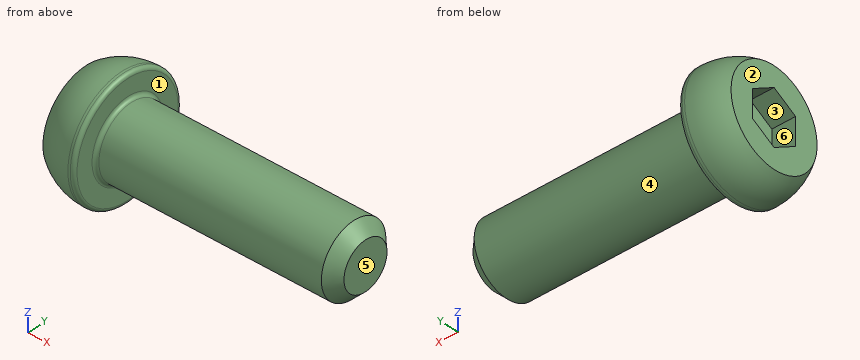
from build123d import *

# Parameters (mm, degrees)
CUT_EXTRUDE_1_DEPTH = 2
FILLET_1_R          = 0.3
CHAMFER_1_SIZE      = 1


with BuildPart() as part:
    # Эскиз1 → Повернуть1 (revolve)
    with BuildSketch(Plane.XY):
        with BuildLine():
            Line((0, 0), (0, 4))
            ThreePointArc((0, 4), (1.41886117, 4.74341649), (3, 5))
            Line((3, 5), (3.5, 5))
            Line((3.5, 5), (3.5, 3))
            Line((3.5, 3), (23.5, 3))
            Line((23.5, 3), (23.5, 0))
            Line((23.5, 0), (0, 0))
        make_face()
    revolve(axis=Axis((23.5, 0, 0), (-1, 0, 0)))

    # Эскиз2 → Вырез-Вытянуть1 (cut)
    with BuildSketch(Plane.ZY):
        Polygon((1.154700538, 2), (-1.154700538, 2), (-2.309401077, 0), (-1.154700538, -2), (1.154700538, -2), (2.309401077, 0), align=None)
    extrude(amount=-CUT_EXTRUDE_1_DEPTH, mode=Mode.SUBTRACT)

    # Скругление1
    fillet_1_edges = [part.edges().sort_by_distance(p)[0] for p in [
        (3.5, -3, 0),
        (3.5, -5, 0),
    ]]
    fillet(fillet_1_edges, radius=FILLET_1_R)

    # Фаска1
    chamfer_1_edges = [part.edges().sort_by_distance(p)[0] for p in [
        (23.5, -3, 0),
    ]]
    chamfer(chamfer_1_edges, length=CHAMFER_1_SIZE)


solid = part.part
Can you work these out from the model? Positions are in its coordinate system, mm. Face numbers are marked on the shaded views. A direction names the side the tool comes from. Coordinates: 2 decimals unless noted, no trailing zeros. Loops run counter-clockwise (first coordinate to the right, second up) from the corner with the lowest first, then second, coordinate; pieces in that order, holes last. Notation, with made-up numbers: (33.25, 62) - (60.25, 62) arc R19 cw to (60.25, 78) - close; hole circle Ø11 at (-33.75, -24). An arc over 180 degrees is marked (long way). Answer as a JSON object with one key per item and string values. Group by question number.
Item 1: On a 3-axis mill with a long thin cutter (end or side, diameter ignored), from which of +Z, -Z, +X, -X, +Y, -Y can I reach the whole of each face in a straight line? I mean the marked faces 1, 2 and 3. Say none if no direction works.
Item 2: If we section it at A-A (z = 0): List the corners of the cut face in (x, y) for me.
Item 3: If I drill on L1, parallel to X at y = -1.5, z = -3; L2, parallel to X at y = 0.5, z = 0; L3, parallel to Y at x = 9, z = 0, over which ranges is the centre line in solid material (lowest first)? Write a range as from..to.
Item 4: If we mould it in two halves opening along Z, with no side actions, what happens to the marked faces 4, 5 and 6? For each: released by +Z, released by -Z, zero draft, split by the parting line, or undercut.
Item 5: For pin 1 (6 mm diameter, centred on x = 8.5, z = -1, fed in from +Y); pin 2 (1.6 mm diameter, centred on x = 0.5, z = 0.5, fed in from -Y); pin 3 (1.6 mm diameter, centred on x = 0.5, z = 0, fed in from +Y), each with a flat end and sliding along its axis, tell me the tip position at first contact or that it passes through.
Item 6: If we section it at B-B (x = 15.75): List the corners of the cut face in (y, z) for me.
Returned:
{
 "1": {"face 1": "+X", "face 2": "+Z, -Z, -X, +Y, -Y", "face 3": "-X"},
 "2": {"outline": "(0, -4) arc R5 ccw to (3, -5) - (3.2, -5) arc R0.3 ccw to (3.5, -4.7) - (3.5, -3.3) arc R0.3 cw to (3.8, -3) - (22.5, -3) - (23.5, -2) - (23.5, 2) - (22.5, 3) - (3.8, 3) arc R0.3 cw to (3.5, 3.3) - (3.5, 4.7) arc R0.3 ccw to (3.2, 5) - (3, 5) arc R5 ccw to (0, 4) - (0, 2) - (2, 2) - (2, -2) - (0, -2) - close"},
 "3": {"L1": "x = 0..3.5", "L2": "x = 2..23.5", "L3": "y = -3..3"},
 "4": {"face 4": "split by the parting line", "face 5": "zero draft", "face 6": "undercut"},
 "5": {"pin 1": "stops at y = 3", "pin 2": "stops at y = -4.68", "pin 3": "stops at y = 4.7"},
 "6": {"outline": "circle Ø6 at (0, 0)"}
}
